Answer from the drawing. Dimensions are ordinates in mm from the lowest x, y and z of the part. Give positions to 0.01 mm unless a question says otherwise; leave off trailing zeros. Loops run counter-clockwise (first coordinate to the right, second up) from the corner with the lowest first, then second, coordinate; pieces in that order, holes last. Notation, with made-up numbers: (26, -22) - (49, -22) arc R23 cw to (49, -11) - close; hole circle Ø1 at (-27.75, 11). An arc over 180 degrees is marked (long way). One line per item, written item: value.
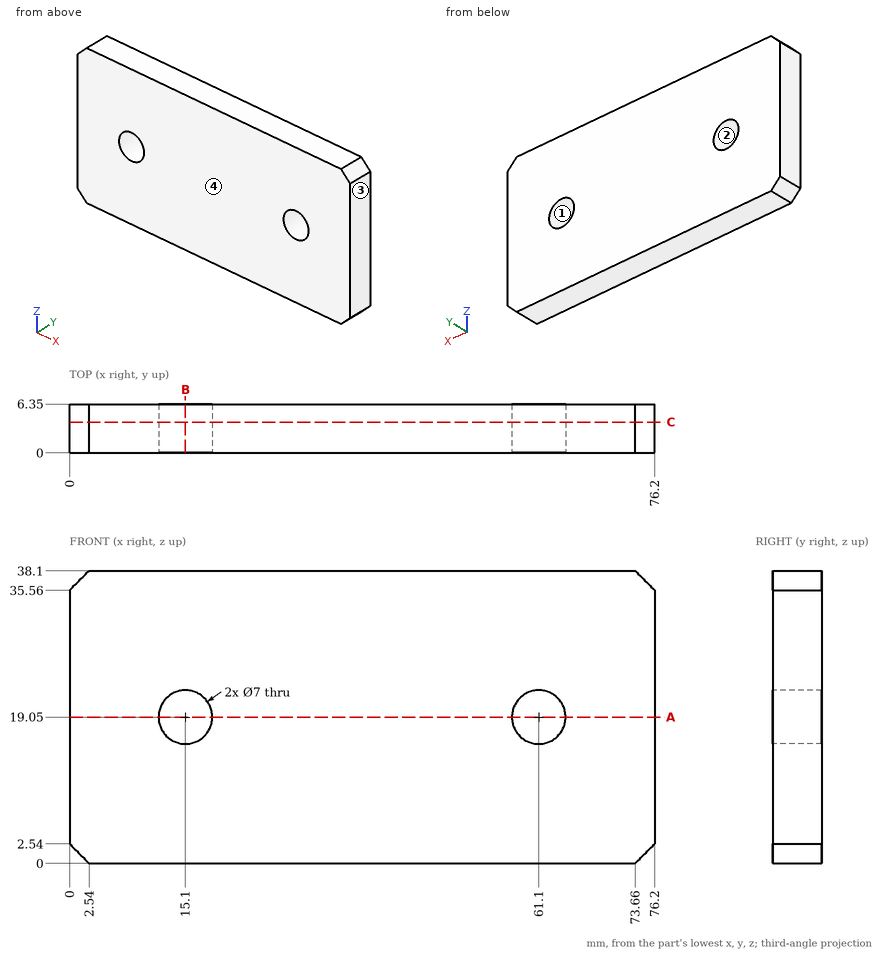
1. Section A-A (z = 19.05) is taken. Write down the section's boundary in (x, y).
Output:
outline: (0, 0) - (11.6, 0) - (11.6, 6.35) - (0, 6.35) - close; (18.6, 0) - (57.6, 0) - (57.6, 6.35) - (18.6, 6.35) - close; (64.6, 0) - (76.2, 0) - (76.2, 6.35) - (64.6, 6.35) - close
2. The mould has two halves that part along X. Classify the marked faces 1, 2, 3 and 4: released by +X, released by -X, zero draft, split by the parting line, or undercut.
Output:
face 1: undercut
face 2: undercut
face 3: released by +X
face 4: zero draft
3. A flat-ended cylindrical pin translates along its axis: pin 1 Ø5.5 at (x, z) = (61.1, 19.05) entering from +Y. Find the tip coordinate at first contact, or state that the pin passes through.
Output:
pin 1: passes through
4. Find the intervals of material crossed by line 1 along Z through (x, y) = (61.1, 2.5); line 2 along X through (y, z) = (1.75, 20); line 3 along Z through (x, y) = (59, 6), in increasing order.
Output:
line 1: z = 0 to 15.55, 22.55 to 38.1
line 2: x = 0 to 11.73, 18.47 to 57.73, 64.47 to 76.2
line 3: z = 0 to 16.25, 21.85 to 38.1
5. Section C-C (y = 4) is taken. Write down the section's boundary in (x, z).
Output:
outline: (0, 2.54) - (2.54, 0) - (73.66, 0) - (76.2, 2.54) - (76.2, 35.56) - (73.66, 38.1) - (2.54, 38.1) - (0, 35.56) - close; hole circle Ø7 at (15.1, 19.05); hole circle Ø7 at (61.1, 19.05)
6. Section B-B (x = 15.1) is taken. Write down the section's boundary in (y, z).
Output:
outline: (0, 0) - (6.35, 0) - (6.35, 15.55) - (0, 15.55) - close; (0, 22.55) - (6.35, 22.55) - (6.35, 38.1) - (0, 38.1) - close
